For this review, use the dimensioned drawing (mm, ordinates from the lowest corner) and the shaded views. Round coordinates to 2 decimals unless told otherwise and drop trailing zeros. Order: outer loops, then holes, each group sorted by start corner. A loop starts at its lowest first (then second) coordinate and runs counter-clockwise, first axis right, second up. Notation, with made-up numbers: (39.5, 25.5) -> (82.5, 25.5) arc R13 ccw to (82.5, 44.5) -> close; hole circle Ø9 at (72, 84). An arc over 180 degrees is marked (long way). Answer in a Markdown table with one row per item.
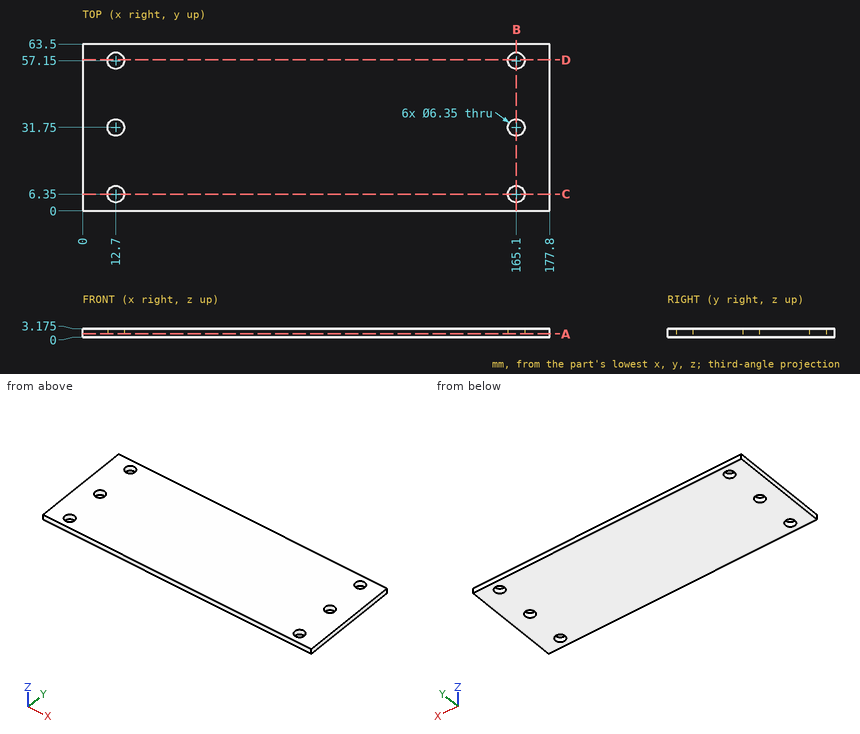
Q1. Clearance check with a flat-ended pin moving along its axis: pin 1 Ø1 at (x, y) = (152.5, 28) entering from -Z. State where the tip first meets the part, or that it passes through.
Answer key:
| item | result |
|---|---|
| pin 1 | stops at z = 0 |
Q2. Take a section at B-B, the plane x = 165.1. Write out the cut boundary in (y, z) (3 decimals), then the cut area to 3 significant figures.
Answer key:
| item | result |
|---|---|
| outline | (0, 0) -> (3.175, 0) -> (3.175, 3.175) -> (0, 3.175) -> close; (9.525, 0) -> (28.575, 0) -> (28.575, 3.175) -> (9.525, 3.175) -> close; (34.925, 0) -> (53.975, 0) -> (53.975, 3.175) -> (34.925, 3.175) -> close; (60.325, 0) -> (63.5, 0) -> (63.5, 3.175) -> (60.325, 3.175) -> close |
| area | 141 mm^2 |
Q3. To check wall thickness, follow probe 1 along Y at (x, z) = (165.1, 2.2) (3 decimals); probe 2 along X at (y, z) = (6.35, 1.2) (3 decimals). State the ranges of each line that lie inside material, in increasing order.
Answer key:
| item | result |
|---|---|
| probe 1 | y = 0 to 3.175, 9.525 to 28.575, 34.925 to 53.975, 60.325 to 63.5 |
| probe 2 | x = 0 to 9.525, 15.875 to 161.925, 168.275 to 177.8 |
Q4. Take a section at D-D, the plane y = 57.5. Write out the cut boundary in (x, z) (3 decimals), then the cut area to 3 significant figures.
Answer key:
| item | result |
|---|---|
| outline | (0, 0) -> (9.544, 0) -> (9.544, 3.175) -> (0, 3.175) -> close; (15.856, 0) -> (161.944, 0) -> (161.944, 3.175) -> (15.856, 3.175) -> close; (168.256, 0) -> (177.8, 0) -> (177.8, 3.175) -> (168.256, 3.175) -> close |
| area | 524 mm^2 |
Q5. Take a section at A-A, the plane z = 1.3. Write out the cut boundary in (x, y) (3 decimals).
Answer key:
| item | result |
|---|---|
| outline | (0, 0) -> (177.8, 0) -> (177.8, 63.5) -> (0, 63.5) -> close; hole circle Ø6.35 at (12.7, 6.35); hole circle Ø6.35 at (12.7, 31.75); hole circle Ø6.35 at (12.7, 57.15); hole circle Ø6.35 at (165.1, 6.35); hole circle Ø6.35 at (165.1, 31.75); hole circle Ø6.35 at (165.1, 57.15) |
Q6. Take a section at C-C, the plane y = 6.35. Write out the cut boundary in (x, z) (3 decimals), then the cut area to 3 significant figures.
Answer key:
| item | result |
|---|---|
| outline | (0, 0) -> (9.525, 0) -> (9.525, 3.175) -> (0, 3.175) -> close; (15.875, 0) -> (161.925, 0) -> (161.925, 3.175) -> (15.875, 3.175) -> close; (168.275, 0) -> (177.8, 0) -> (177.8, 3.175) -> (168.275, 3.175) -> close |
| area | 524 mm^2 |
